```python
from build123d import *

# Parameters (mm, degrees)
F1_DEPTH = 50.8


with BuildPart() as f1:
    # F0 (on Front) → F1 (new body)
    with BuildSketch(Plane.XZ):
        with BuildLine():
            ThreePointArc((-17.360634, -0.82199), (-23.884981, 5.155183), (-30.049838, -1.192117))
            Line((-30.049838, -1.192117), (-30.049838, -36.133546))
            Line((-30.049838, -36.133546), (34.392419, -36.133546))
            ThreePointArc((34.392419, -36.133546), (38.882547, -34.273674), (40.742419, -29.783546))
            Line((40.742419, -29.783546), (40.742419, -23.495))
            ThreePointArc((40.742419, -23.495), (38.882547, -19.004872), (34.392419, -17.145))
            Line((34.392419, -17.145), (-16.407581, -17.145))
            Line((-16.407581, -17.145), (-17.360634, -0.82199))
        make_face()
    extrude(amount=F1_DEPTH)


solid = f1.part
```
For this review, take the finished solid that the model builds, in its own axes (mm). A direction names the side the tool comes from. Give positions to 0.01 mm unless a question says otherwise; leave off trailing zeros. Write each loop counter-clockwise with the first axis right and the second up, starting at its lowest first coordinate (ties: lowest second). Pieces come first, ordered by that corner, then holes.
Item 1: Take a section at A-A (y = -47). Give the boundary of the cut face in (x, z) (3 decimals).
Item 2: Take a section at C-C (z = -11). Give the boundary of the cut face in (x, y).
Item 3: Insertion check: P1, Ø4, axis at x = 21, y = -9, coming from the +Z side (3 decimals); P2, Ø10, axis at x = -18, y = -45, coming from the +Z side; P3, Ø1.5, axis at x = -19.5, z = -27, coming from the +Y side; P4, Ø4, axis at y = -41, z = -19, coming from the +X side. Each pin has a flat end and moves straight along its axis. Give the tip position at first contact, or say it passes through.
Item 4: Wall thickness on probe 1 along Z at (x, y) = (24, -6.5) (3 decimals); probe 2 along X at (y, z) = (-10.5, -17); probe 3 along X at (y, z) = (-12.5, -10): over which ranges is each line inside the solid? List them lowest first.
Item 5: Machinability: for faces 1 (the face through (9, -25, -17.145)), 2 (the face through (40.742, -25, -27)), which of the approach directions +Z, -Z, +X, -X, +Y, -Y give a long, thin tool a straight path to every point of the face, cutting with its end or side? Answer none if there is none.
Item 6: Take a section at B-B (x = 21). Give the boundary of the cut face in (y, z) (3 decimals).
Established:
1. outline: (-30.05, -36.134) - (34.392, -36.134) arc R6.35 ccw to (40.742, -29.784) - (40.742, -23.495) arc R6.35 ccw to (34.392, -17.145) - (-16.408, -17.145) - (-17.361, -0.822) arc R6.35 ccw to (-30.05, -1.192) - close
2. outline: (-30.05, -50.8) - (-16.77, -50.8) - (-16.77, 0) - (-30.05, 0) - close
3. P1: stops at z = -17.145
3. P2: stops at z = 5.12
3. P3: stops at y = 0
3. P4: stops at x = 40.23
4. probe 1: z = -36.134 to -17.145
4. probe 2: x = -30.05 to -16.42
4. probe 3: x = -30.05 to -16.82
5. face 1: +Z, +X, +Y, -Y
5. face 2: +Z, -Z, +X, +Y, -Y
6. outline: (-50.8, -36.134) - (0, -36.134) - (0, -17.145) - (-50.8, -17.145) - close
